Source: three-view drawing plus pictorial views. Frame: mm from the lowest corner of the part. A direction names the side the tool comes from. Give positions to 0.01 mm unless a question says otherwise; leave off trailing zeros. Order: outer loops, then holes, each group sorted by start corner. A loop starts at its lowest first (then second) coordinate and runs counter-clockwise, first axis right, second up.
1) Access query for the marked faces 1 and 2. Directions: +Z, -Z, +X, -X, +Y, -Y. A direction counts if a zero-diameter tool reaches every point of the face in a straight line with its end or side. Return the directions, or none.
2) Material intervals for line 1 (Z direction, x = 60, y = 15) (1 decimal); line 2 (X direction, y = 5, z = 27); line 3 (Y direction, x = 88, z = 19.5), sorted ascending.
3) Section D-D, the plane z = 14. Return loops of the section in (x, y) (1 decimal), plus the area to 3 significant figures.
4) Section A-A, the plane y = 17. Return loops of the section in (x, z) (1 decimal), plus the area to 3 significant figures.
5) First-contact query: P1, Ø6, axis at x = 82.5, z = 21.5, coming from the -Y side; P2, Ø3, axis at x = 77.5, z = 28.5, coming from the -Y side; P3, Ø0.9, axis at x = 105, y = 30.5, coming from the -Z side (1 decimal). Flat tips, straight axial feed; report the tip coordinate or a pass-through.
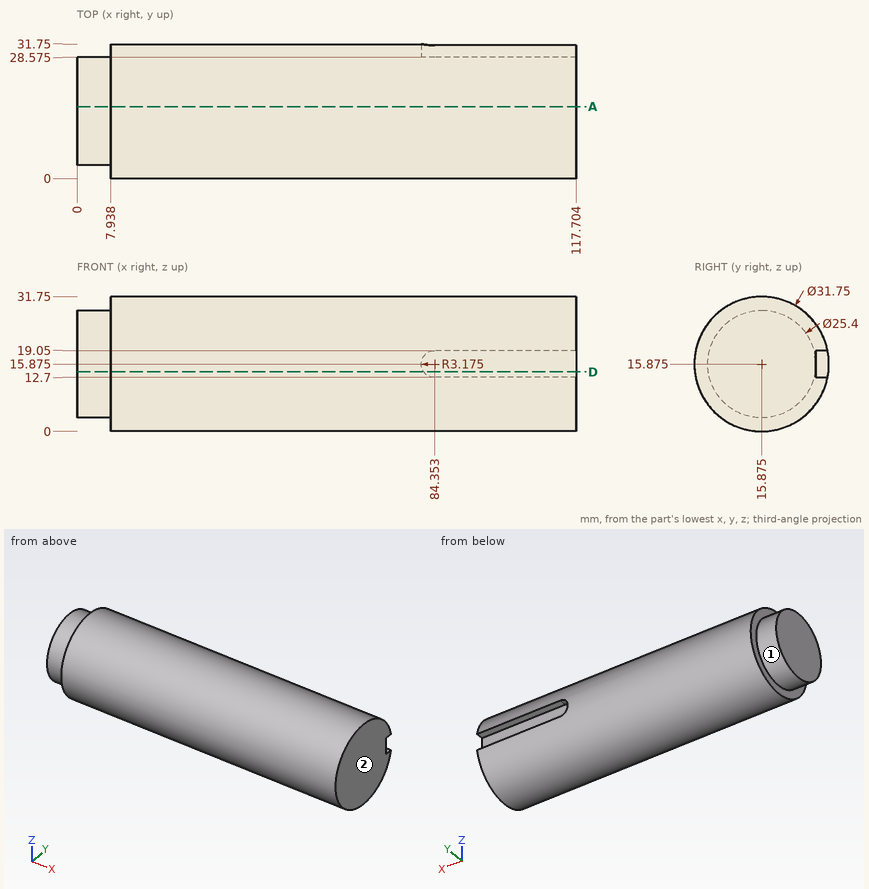
From the geometry:
1. face 1: -X
1. face 2: +Z, -Z, +X, +Y, -Y
2. line 1: z = 0 to 31.7
2. line 2: x = 7.94 to 117.7
2. line 3: y = 0.42 to 31.33
3. outline: (0, 3.3) - (7.9, 3.3) - (7.9, 0.1) - (117.7, 0.1) - (117.7, 28.6) - (81.8, 28.6) - (81.8, 31.6) - (7.9, 31.6) - (7.9, 28.4) - (0, 28.4) - close
3. area: 3,550 mm2
4. outline: (0, 3.2) - (7.9, 3.2) - (7.9, 0) - (117.7, 0) - (117.7, 31.7) - (7.9, 31.7) - (7.9, 28.5) - (0, 28.5) - close
4. area: 3,680 mm2
5. P1: stops at y = 0.22
5. P2: stops at y = 4.55
5. P3: stops at z = 8.7
